```python
from build123d import *

# Parameters (mm, degrees)
SKETCH1_R           = 30
BOSS_EXTRUDE1_DEPTH = 26
BOSS_EXTRUDE2_DEPTH = 250
SKETCH3_R           = 13
CUT_EXTRUDE1_DEPTH  = 26
SKETCH1_2_R         = 30
CUT_EXTRUDE2_DEPTH  = 8
SKETCH4_R           = 19
CUT_EXTRUDE3_DEPTH  = 210
SKETCH6_R           = 19
SKETCH6_R_2         = 18
BOSS_EXTRUDE3_DEPTH = 10
SKETCH7_W           = 4
SKETCH7_H           = 4
BOSS_EXTRUDE4_DEPTH = 26
CUT_EXTRUDE4_REACH  = 262.998


with BuildPart() as part:
    # Sketch1 → Boss-Extrude1 (new, symmetric)
    with BuildSketch(Plane(origin=(0, 0, 0), x_dir=(1, 0, 0), z_dir=(0, 1, 0))):
        with Locations(Location((0, 0, 0), (0, 0, 90))):
            Circle(SKETCH1_R)
    extrude(amount=BOSS_EXTRUDE1_DEPTH, both=True)

    # Sketch2 → Boss-Extrude2 (add)
    with BuildSketch(Plane.XY):
        with BuildLine():
            Line((30, 26), (30, -26))
            Line((30, -26), (26, -26))
            Line((26, -26), (26, -23))
            Line((26, -23), (-2, -23))
            ThreePointArc((-2, -23), (-25, 0), (-2, 23))
            Line((-2, 23), (26, 23))
            Line((26, 23), (26, 26))
            Line((26, 26), (30, 26))
        make_face()
    extrude(amount=BOSS_EXTRUDE2_DEPTH)

    # Sketch3 → Cut-Extrude1 (cut, symmetric)
    with BuildSketch(Plane(origin=(0, 0, 0), x_dir=(1, 0, 0), z_dir=(0, 1, 0))):
        with Locations(Location((0, 0, 0), (0, 0, 270))):
            Circle(SKETCH3_R)
    extrude(amount=CUT_EXTRUDE1_DEPTH, both=True, mode=Mode.SUBTRACT)

    # Sketch1<2> → Cut-Extrude2 (cut, symmetric)
    with BuildSketch(Plane(origin=(0, 0, 0), x_dir=(1, 0, 0), z_dir=(0, 1, 0))):
        Circle(SKETCH1_2_R)
    extrude(amount=CUT_EXTRUDE2_DEPTH, both=True, mode=Mode.SUBTRACT)

    # Sketch4 → Cut-Extrude3 (cut)
    with BuildSketch(Plane.XY.offset(250)):
        Circle(SKETCH4_R)
    extrude(amount=-CUT_EXTRUDE3_DEPTH, mode=Mode.SUBTRACT)

    # Sketch6 → Boss-Extrude3 (add)
    with BuildSketch(Plane.XY.offset(250)):
        Circle(SKETCH6_R)
        Circle(SKETCH6_R_2, mode=Mode.SUBTRACT)
    extrude(amount=-BOSS_EXTRUDE3_DEPTH)

    # Sketch7 → Boss-Extrude4 (add, symmetric)
    with BuildSketch(Plane(origin=(0, 0, 0), x_dir=(1, 0, 0), z_dir=(0, 1, 0))):
        with Locations((28, -252)):
            Rectangle(SKETCH7_W, SKETCH7_H)
    extrude(amount=BOSS_EXTRUDE4_DEPTH, both=True)

    # Cut-Extrude4: up to this face of the body (flat: up to its plane)
    cut_extrude4_end = Plane(part.part.faces().sort_by_distance((28.902688409, -26, 134.483314774))[0])
    # Sketch9 → Cut-Extrude4 (cut, up to the picked face)
    with BuildSketch(Plane(origin=(0, 26, 0), x_dir=(1, 0, 0), z_dir=(0, 1, 0)), mode=Mode.PRIVATE) as cut_extrude4_sk1:
        with BuildLine():
            Line((-23.273636947, 18.92981308), (-10.085242677, 8.202919002))
            ThreePointArc((-10.085242677, 8.202919002), (0.632804436, 12.984589271), (10.835093825, 7.183365632))
            Line((10.835093825, 7.183365632), (22.960343515, 19.308615323))
            ThreePointArc((22.960343515, 19.308615323), (-0.245786449, 29.998993133), (-23.273636947, 18.92981308))
        make_face()
    cut_extrude4_tool1 = split(extrude(cut_extrude4_sk1.sketch, amount=-CUT_EXTRUDE4_REACH, mode=Mode.PRIVATE), bisect_by=cut_extrude4_end, keep=Keep.BOTH, mode=Mode.PRIVATE)
    add(cut_extrude4_tool1.solids().sort_by(Axis((0.119463, 26, -19.65599), (0, -1, 0)))[0], mode=Mode.SUBTRACT)


solid = part.part
```
Geometry check sheet. Reference: the model listing, model coordinates, mm. A direction names the side the tool comes from. Give positions to 0.01 mm unless a question says otherwise; leave off trailing zeros. Loops run counter-clockwise (first coordinate to the right, second up) from the corner with the lowest first, then second, coordinate; pieces in that order, holes last. Notation, with made-up numbers: M 62.25,20.5 L 89.25,20.5 A9 ccw 89.25,34.5 Z; hole C 5,-39.5 d10. An arc over 180 degrees is marked long. Write item = value, one per line. Start each with the question number.
1. Draft check along Z on faces 4 (the face through (30, 0, 129)), 5 (the face through (-1.03, -16.87, 12.96)), 6 (the face through (16.81, -16.87, -13.16)). Enter one of: +Z half, -Z half, draft (parallel to the pull), parting line (faces both ways), or undercut.
2. Section check D-D, the plane x = 8. Enter the section's corners in (y, z), plus the area to 3 significant figures.
3. Section check C-C, the plane z = 109.5. Enter the section's corners in (x, y).
4. Section check A-A, the plane y = 0. Enter the section's corners in (x, z).
5. Go/stop test with flat-tipped pins: P1, Ø8.5, axis at x = 16, z = 140.5, coming from the +Y side; P2, Ø14, axis at x = 10, z = 75.5, coming from the -Y side; P3, Ø15.5, axis at y = -8, z = 148, coming from the -X side; P4, Ø21, axis at x = 0, z = 0, coming from the -Y side. Record where each tip stops, or that it passes through.
6. Tool access check on faces 1 (the face through (16.81, 17.13, -13.16)), 2 (the face through (8.145, 0.112, 28.873)), 3 (the face through (-24.994, -0.506, 131.658)). Record the directions out of +Z, -Z, +X, -X, +Y, -Y that give a thin tool (end or side, any length) a straight path to the whole face; none if there is none.
7. Section check B-B, the plane z = 6. Enter the section's corners in (x, y).
8. Thickness scan on probe 1 along Y at (x, z) = (14, 4.5); probe 2 along X at (y, z) = (-17, 0); probe 3 along Z at (x, y) = (0, -16.5). Record the ranges inside material, lowest first.
Values follow:
q1.face_4 = draft
q1.face_5 = undercut
q1.face_6 = -Z half
q2.outline = M -26,10.25 L -8,10.25 L -8,28.91 L 8,28.91 L 8,10.25 L 26,10.25 L 26,28.91 L 23,28.91 L 23,250 L 16.12,250 L 16.12,240 L 17.23,240 L 17.23,40 L -17.23,40 L -17.23,240 L -16.12,240 L -16.12,250 L -23,250 L -23,28.91 L -26,28.91 Z
q2.area = 3,630 mm^2
q3.outline = M -2,-23 L 26,-23 L 26,-26 L 30,-26 L 30,26 L 26,26 L 26,23 L -2,23 A23 ccw Z; hole C 0,0 d38
q4.outline = M -25,16.58 A30 cw 30,0 L 30,254 L 26,254 L 26,250 L 18,250 L 18,240 L 19,240 L 19,40 L -19,40 L -19,240 L -18,240 L -18,250 L -25,250 Z
q5.P1 = 23
q5.P2 = -23
q5.P3 = -25
q5.P4 = through
q6.face_1 = -Z, +Y, -Y
q6.face_2 = -Z
q6.face_3 = +Z, -X
q7.outline = M -29.39,-26 L -11.53,-26 L -11.53,-8 L -29.39,-8 Z; M -29.39,8 L -11.53,8 L -11.53,26 L -29.39,26 Z; M 11.53,-26 L 30,-26 L 30,26 L 11.53,26 L 11.53,8 L 29.39,8 L 29.39,-8 L 11.53,-8 Z
q8.probe_1 = -26 to -8, 8 to 26
q8.probe_2 = -30 to -13, 13 to 30
q8.probe_3 = 13 to 40
